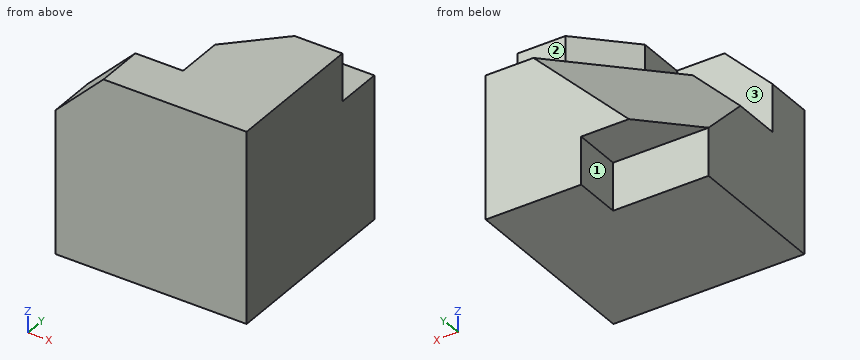
from build123d import *

# Parameters (mm, degrees)
BOSS_EXTRUDE1_DEPTH = 20
BOSS_EXTRUDE2_DEPTH = 20
CUT_EXTRUDE1_DEPTH  = 20
BOSS_EXTRUDE3_DEPTH = 5
BOSS_EXTRUDE4_DEPTH = 5
SKETCH7_W           = 5
SKETCH7_H           = 15
BOSS_EXTRUDE5_DEPTH = 10


with BuildPart() as part:
    # Sketch2 → Boss-Extrude1 (new body)
    with BuildSketch(Plane(origin=(0, 0, 0), x_dir=(1, 0, 0), z_dir=(0, 1, 0))):
        Polygon((-10, -5), (-10, 0), (0, 0), (0, -15), (-5, -15), (-15, -5), align=None)
    extrude(amount=BOSS_EXTRUDE1_DEPTH)

    # Sketch3 → Boss-Extrude2 (add)
    with BuildSketch(Plane(origin=(0, 0, 0), x_dir=(-1, 0, 0), z_dir=(0, -1, 0))):
        Polygon((15, -5), (5, -15), (15, -15), (20, -10), (20, -5), align=None)
    extrude(amount=-BOSS_EXTRUDE2_DEPTH)

    # 3DSketch2 → Cut-Extrude1 (cut, along a direction that is not the sketch's normal)
    with BuildSketch(Plane(origin=(-15, 20, 5), x_dir=(0, -0.7071067811865476, 0.7071067811865475), z_dir=(-0.5773502691896257, 0.5773502691896257, 0.5773502691896257))):
        Polygon((0, 0), (7.071067812, 12.247448714), (14.142135624, 0), (10.606601718, -6.123724357), (3.535533906, -6.123724357), align=None)
    extrude(amount=CUT_EXTRUDE1_DEPTH, dir=(0, 1, 0), mode=Mode.SUBTRACT)

    # Sketch5 → Boss-Extrude3 (add)
    with BuildSketch(Plane.XY.offset(15)):
        Polygon((0, 15), (-5, 15), (-10, 10), (-10, 5), (-15, 5), (-15, 0), (0, 0), align=None)
    extrude(amount=BOSS_EXTRUDE3_DEPTH)

    # Sketch6 → Boss-Extrude4 (add)
    with BuildSketch(Plane(origin=(0, 0, 0), x_dir=(-1, 0, 0), z_dir=(0, -1, 0))):
        Polygon((20, -10), (15, -15), (15, -20), (20, -15), align=None)
    extrude(amount=-BOSS_EXTRUDE4_DEPTH)

    # Sketch7 → Boss-Extrude5 (add)
    with BuildSketch(Plane.ZY.offset(10)):
        with Locations((2.5, 7.5)):
            Rectangle(SKETCH7_W, SKETCH7_H)
    extrude(amount=BOSS_EXTRUDE5_DEPTH)


solid = part.part
Part model, mm, in its own coordinate system. Face numbers are marked on the shaded views. A direction names the side the tool comes from. Round coordinates to 2 decimals unless told otherwise and drop trailing zeros. Loops run counter-clockwise (first coordinate to the right, second up) from the corner with the lowest first, then second, coordinate; pieces in that order, holes last. Notation, with made-up numbers: (81, 65) - (122, 65) arc R14 ccw to (122, 69) - close; hole circle Ø7 at (-11, 9.25). An arc over 180 degrees is marked (long way). Answer as a JSON object with one key per item and string values.
Item 1: Tool access for the marked faces 1, 2 and 3: list every direction of +Z, -Z, +X, -X, +Y, -Y with a clear straight run to the whole face (end or side of a thin tool).
Output:
{"face 1": "-Z, -X, +Y", "face 2": "+Z, +X, -X, +Y", "face 3": "+Z, -X, +Y"}
Item 2: Band-saw the part on B-B on z = 18.25. List the corners of the cut face in (x, y).
Output:
{"outline": "(-16.75, 0) - (0, 0) - (0, 15) - (-5, 15) - (-10, 10) - (-10, 5) - (-16.75, 5) - close"}
Item 3: Band-saw the part on D-D on z = 4.25. List the corners of the cut face in (x, y), plus the area to 3 significant figures.
Output:
{"outline": "(-20, 0) - (0, 0) - (0, 20) - (-10, 20) - (-10, 15) - (-20, 15) - close", "area": "350 mm2"}
Item 4: Band-saw the part on A-A on y = 10.5. List the corners of the cut face in (x, z), plus the area to 3 significant figures.
Output:
{"outline": "(-20, 0) - (0, 0) - (0, 20) - (-9.5, 20) - (-9.5, 15) - (-14.5, 15) - (-20, 9.5) - close", "area": "332 mm2"}
Item 5: Pin check, flat tips, straight feed: pin 1 (6 mm diameter, centred on x = -14.5, y = 12.5, fed in from +Z); pin 2 (4 mm diameter, centred on y = 6.5, z = 18, fed in from -X); pin 3 (1.5 mm diameter, centred on y = 18.5, z = 1.5, fed in from -X). Stop position of each tip, or through.
Output:
{"pin 1": "z = 15", "pin 2": "x = -18.32", "pin 3": "x = -10"}
Item 6: Wall check: L1, parallel to Y at x = -10.75, z = 16.5; L2, parallel to X at y = 15.75, z = 3; L3, parallel to Y at x = -13.75, z = 4. Give the ranges that are in metal, low to high.
Output:
{"L1": "0 to 5", "L2": "-10 to 0", "L3": "0 to 15"}
Item 7: Band-saw the part on C-C on x = -11.5. List the corners of the cut face in (y, z).
Output:
{"outline": "(0, 0) - (15, 0) - (15, 5) - (20, 5) - (20, 8.5) - (13.5, 15) - (5, 15) - (5, 20) - (0, 20) - close"}
